Autodesk Inventor part; units mm, degrees
ref_plane "YZ Plane" through (0, 0, 0) normal (1, 0, 0) x (0, 1, 0)
ref_plane "XZ Plane" through (0, 0, 0) normal (0, 1, 0) x (-1, 0, 0)
ref_plane "XY Plane" through (0, 0, 0) normal (0, 0, 1) x (1, 0, 0)
sketch "草圖1" plane through (0, 0, 0) normal (0, 0, 1) x (1, 0, 0)
  line L0 (0, 0) -> (-25.6572, 0) construction
  line L1 (0, 0) -> (0, 25.6407) construction
  line L2 (-23.5, -5.5) -> (-13.1185, -5.5)
  line L3 (25, -4) -> (25, 5.5)
  line L4 (25, 5.5) -> (-25, 5.5)
  line L5 (-25, 5.5) -> (-25, -4)
  line L6 (-25, -5.5) -> (25, 5.5) construction
  line L7 (25, -5.5) -> (-25, 5.5) construction
  arc A0 (23.5, -5.5) -> (25, -4) centre (23.5, -4) ccw
  arc A1 (-25, -4) -> (-23.5, -5.5) centre (-23.5, -4) ccw
  line L8 (-13.1185, -5.5) -> (23.5, -5.5)
  line L9 (7.5, 5.5) -> (7.5, 7.5)
  line L10 (7.5, 7.5) -> (-7.5, 7.5)
  line L11 (-7.5, 7.5) -> (-7.5, 5.5)
  circle A2 centre (0, -0.5) radius 3
  dimension "d0" = 50
  dimension "d4" = 1.5
  dimension "d13" = 2
  dimension "d14" = 15
  dimension "d15" = 6
  dimension "d16" = 6
  dimension "d17" = 5
extrude "擠出1" add sketch "草圖1" along normal mid plane 2
equation "\"d4\" = d5"
equation "\"折彎半徑\" = 厚度"
equation "\"折彎離隙寬度\" = 厚度"
equation "\"折彎離隙深度\" = 0.5 * 厚度"
equation "\"最小剩餘\" = 2 * 厚度"
equation "\"轉移半徑\" = 折彎半徑"
equation "\"Jacobi半徑大小\" = 折彎半徑"
equation "\"間隙大小\" = 厚度"
properties part number "0 零件" material "不鏽鋼"
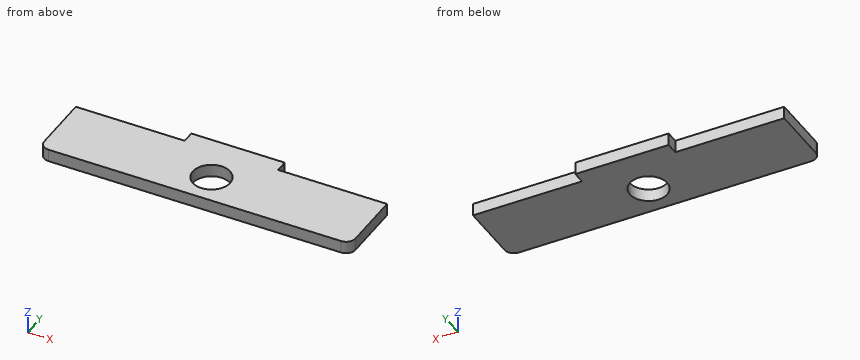
Could you check a few things on this model? Use its own coordinates, in mm. Round coordinates to 2 decimals unless told otherwise and drop trailing zeros. Loops run counter-clockwise (first coordinate to the right, second up) from the corner with the lowest first, then second, coordinate; pieces in that order, holes last. Notation, with made-up numbers: M 6.5,-40 L 59.5,-40 A33 ccw 59.5,-1 Z; hole C -20,14 d8. An arc over 180 degrees is marked long. Put each result on its own line as item: value.
Q1. Imagine slicing it at B-B (z = -0.35). Write out the boundary of the cut face in (x, y).
Check result:
outline: M -25,-4 A1.5 ccw -23.5,-5.5 L 23.5,-5.5 A1.5 ccw 25,-4 L 25,5.5 L 7.5,5.5 L 7.5,7.5 L -7.5,7.5 L -7.5,5.5 L -25,5.5 Z; hole C 0,-0.5 d6
Q2. Imagine slicing it at D-D (x = -12.5). Write out the boundary of the cut face in (y, z).
Check result:
outline: M -5.5,-1 L 5.5,-1 L 5.5,1 L -5.5,1 Z
Q3. Imagine slicing it at C-C (x = 0). Write out the boundary of the cut face in (y, z), then the cut area to 3 significant figures.
Check result:
outline: M -5.5,-1 L -3.5,-1 L -3.5,1 L -5.5,1 Z; M 2.5,-1 L 7.5,-1 L 7.5,1 L 2.5,1 Z
area: 14.0 mm2
Q4. I need wall thicknesses on probe 1 along Y at (x, z) = (0, -0.1); probe 2 along Y at (x, z) = (-19.5, -0.15); probe 3 along X at (y, z) = (7, 0.2). Which ranges of each line are inside material? Lowest first, please.
Check result:
probe 1: -5.5 to -3.5, 2.5 to 7.5
probe 2: -5.5 to 5.5
probe 3: -7.5 to 7.5
Q5. Imagine slicing it at A-A (y = -0.5). Write out the boundary of the cut face in (x, z), then the cut area to 3 significant figures.
Check result:
outline: M -25,-1 L -3,-1 L -3,1 L -25,1 Z; M 3,-1 L 25,-1 L 25,1 L 3,1 Z
area: 88.0 mm2
Q6. For pin 1 (0.6 mm diameter, centred on y = 6, z = -0.5, fed in from -X), with a flat end and sliding along its axis, tell me the tip position at first contact or that it passes through.
Check result:
pin 1: x = -7.5
